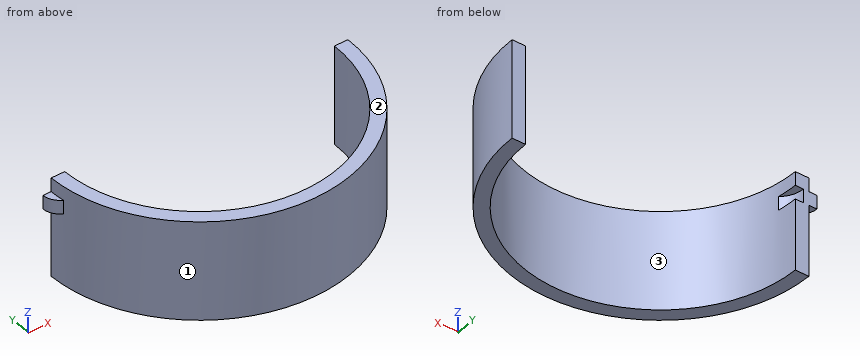
```python
from build123d import *

# Parameters (mm, degrees)
BOSS_EXTRUDE1_DEPTH = 9.144
BOSS_EXTRUDE2_DEPTH = 1.27
CUT_EXTRUDE2_DEPTH  = 1.27


with BuildPart() as part:
    # Sketch1 → Boss-Extrude1 (new body)
    with BuildSketch(Plane.XY):
        with BuildLine():
            Line((13.8938, 13.8938), (12.6238, 13.8938))
            ThreePointArc((12.6238, 13.8938), (0, 1.27), (-12.6238, 13.8938))
            Line((-12.6238, 13.8938), (-13.8938, 13.8938))
            ThreePointArc((-13.8938, 13.8938), (0, 0), (13.8938, 13.8938))
        make_face()
    extrude(amount=-BOSS_EXTRUDE1_DEPTH)

    # Sketch3 → Boss-Extrude2 (add)
    with BuildSketch(Plane.XY.offset(-1.27)):
        with BuildLine():
            Line((-13.8938, 13.8938), (-14.6558, 13.8938))
            ThreePointArc((-14.6558, 13.8938), (-14.431944467, 13.081702502), (-13.82361054, 12.498998908))
            ThreePointArc((-13.82361054, 12.498998908), (-13.87624154, 13.19551699), (-13.8938, 13.8938))
        make_face()
    extrude(amount=-BOSS_EXTRUDE2_DEPTH)

    # Sketch4 → Cut-Extrude2 (cut)
    with BuildSketch(Plane.XY.offset(-1.27)):
        with BuildLine():
            Line((-13.3858, 13.8938), (-12.6238, 13.8938))
            ThreePointArc((-12.6238, 13.8938), (-12.588918043, 12.955999941), (-12.484464942, 12.023382522))
            ThreePointArc((-12.484464942, 12.023382522), (-13.148713609, 12.855668695), (-13.3858, 13.8938))
        make_face()
    extrude(amount=-CUT_EXTRUDE2_DEPTH, mode=Mode.SUBTRACT)


solid = part.part
```
The model under review builds one solid part; all positions refer to its coordinate system, in mm. Face numbers are marked on the shaded views. Round coordinates to 2 decimals unless told otherwise and drop trailing zeros. Loops run counter-clockwise (first coordinate to the right, second up) from the corner with the lowest first, then second, coordinate; pieces in that order, holes last. Notation, with made-up numbers: (61, -24.5) - (78, -24.5) arc R16 cw to (78, -12.5) - close; hole circle Ø6 at (43, 54.25). An arc over 180 degrees is marked (long way). Write each question's results on one line, items separated by ' | '. Start each with the question number.
Q1. Take a section at C-C on x = 0. Give the boundary of the cut face in (y, z).
Q2. Take a section at A-A on y = 6.25. Give the boundary of the cut face in (x, z).
Q3. Draft analysis for pull direction X (two halves, no side actions). For the marked faces 1, 2 and 3, state which applies: pulls with the +X half, pulls with the -X half, needs draft (parallel to the pull), parting line crosses it, or undercut.
Q4. Wall thickness on line 1 along X through (y, z) = (7.75, -5); line 2 along X through (y, z) = (7.5, -0.25); line 3 along Y through (x, z) = (-1, -0.25): over which ranges is each line inside the solid? List them lowest first. Write a range as [from, to].
Q5. Take a section at B-B on y = 4.25. Give the boundary of the cut face in (x, z).
Q6. Take a section at D-D on z = -4. Give the boundary of the cut face in (x, y), plus the area to 3 significant figures.
Q7. Insertion check: P1, Ø0.5, axis at x = -13, y = 13, coming from the +Z side; P2, Ø4, axis at y = 2, z = -5.5, coming from the +X side; P3, Ø1.5, axis at x = 9.5, z = -3, coming from the +Y side; P4, Ø8, axis at x = 2.5, y = 6.5, coming from the +Z side. Each pin has a flat end and moves straight along its axis. Give the tip position at first contact, or say it passes through.
Data:
1) outline: (0, -9.14) - (1.27, -9.14) - (1.27, 0) - (0, 0) - close
2) outline: (-11.6, -9.14) - (-10.05, -9.14) - (-10.05, 0) - (-11.6, 0) - close; (10.05, -9.14) - (11.6, -9.14) - (11.6, 0) - (10.05, 0) - close
3) face 1: parting line crosses it | face 2: needs draft | face 3: undercut
4) line 1: x = [-12.46, -11.03], [11.03, 12.46] | line 2: x = [-12.34, -10.88], [10.88, 12.34] | line 3: y = [0.04, 1.31]
5) outline: (-10, -9.14) - (-8.15, -9.14) - (-8.15, 0) - (-10, 0) - close; (8.15, -9.14) - (10, -9.14) - (10, 0) - (8.15, 0) - close
6) outline: (-13.89, 13.89) arc R13.89 ccw to (13.89, 13.89) - (12.62, 13.89) arc R12.62 cw to (-12.62, 13.89) - close | area: 52.9 mm²
7) P1: stops at z = 0 | P2: stops at x = 9.75 | P3: stops at y = 6.53 | P4: passes through
